from build123d import *

# Parameters (mm, degrees)
SKETCH1_R           = 14
SKETCH1_R_2         = 1.5
BOSS_EXTRUDE1_DEPTH = 8
SKETCH2_W           = 5.1
SKETCH2_H           = 3.455751918
CUT_EXTRUDE2_DEPTH  = 9
CIRPATTERN1_COUNT   = 12
BOSS_EXTRUDE2_START = -4
SKETCH3_R           = 5
SKETCH3_R_2         = 1.5
BOSS_EXTRUDE2_DEPTH = 4


with BuildPart() as part:
    # Sketch1 → Boss-Extrude1 (new body)
    with BuildSketch(Plane.XY):
        Circle(SKETCH1_R)
        Circle(SKETCH1_R_2, mode=Mode.SUBTRACT)
    extrude(amount=BOSS_EXTRUDE1_DEPTH)

    # Sketch2 → Cut-Extrude2 (cut)
    with BuildSketch(Plane.XY):
        with Locations((11.75, 0)):
            Rectangle(SKETCH2_W, SKETCH2_H)
    cut_extrude2 = extrude(amount=CUT_EXTRUDE2_DEPTH, mode=Mode.SUBTRACT)

    # CirPattern1: Cut-Extrude2 ×12 about axis
    cirpattern1_axis = Axis((0, 0, 0), (0, 0, 1))
    for i in range(1, CIRPATTERN1_COUNT):
        add(cut_extrude2.rotate(cirpattern1_axis, i * 360 / CIRPATTERN1_COUNT), mode=Mode.SUBTRACT)

    # Sketch3 → Boss-Extrude2 (add)
    with BuildSketch(Plane.XY.offset(BOSS_EXTRUDE2_START)):
        Circle(SKETCH3_R)
        Circle(SKETCH3_R_2, mode=Mode.SUBTRACT)
    extrude(amount=BOSS_EXTRUDE2_DEPTH)


solid = part.part
Design review of the part built by this model. Coordinates are the model's own, in mm. A direction names the side the tool comes from. Coordinates: 2 decimals unless noted, no trailing zeros. Write each loop counter-clockwise with the first axis right and the second up, starting at its lowest first coordinate (ties: lowest second). Pieces come first, ordered by that corner, then holes. Notation, with made-up numbers: (61, -37.5) - (105, -37.5) arc R9 cw to (105, -31.5) - close; hole circle Ø6 at (88.5, 71). An arc over 180 degrees is marked (long way). One line per item, written item: value.
1) Insertion check: pin 1 (1.7 mm diameter, centred on y = 0, z = 4, fed in from +X); pin 2 (4 mm diameter, centred on x = -0.5, z = 6, fed in from +Y); pin 3 (12 mm diameter, centred on x = 2, y = 8.5, fed in from -Z); pin 4 (1.4 mm diameter, centred on x = -10.5, z = 5, fed in from +Y). Each pin has a flat end and moves straight along its axis. Give the tip position at first contact, or say it passes through.
Answer sheet:
pin 1: stops at x = 9.2
pin 2: stops at y = 13.89
pin 3: stops at z = -4
pin 4: stops at y = 10
2) Add section A-A (y = 0). State the section outline as (x, z) points.
Answer sheet:
outline: (-9.2, 0) - (-5, 0) - (-5, -4) - (-1.5, -4) - (-1.5, 8) - (-9.2, 8) - close; (1.5, -4) - (5, -4) - (5, 0) - (9.2, 0) - (9.2, 8) - (1.5, 8) - close
3) To check wall thickness, follow probe 1 along Y at (x, z) = (4.75, 6.5); probe 2 along Y at (x, z) = (10.5, 3); probe 3 along Y at (x, z) = (5.25, 1.75). State the ranges of each line that lie inside material, in increasing order.
Answer sheet:
probe 1: y = -13.17 to -11.68, -7.88 to 7.88, 11.68 to 13.17
probe 2: y = -9.26 to -8.06, -4.07 to -1.73, 1.73 to 4.07, 8.06 to 9.26
probe 3: y = -12.98 to -12.55, -7.59 to 7.59, 12.55 to 12.98
4) Add section D-D (x = -8). State the section outline as (y, z) points, plus the area to 3 significant figures.
Answer sheet:
outline: (-10.4, 0) - (-6.61, 0) - (-6.61, 8) - (-10.4, 8) - close; (-4.54, 0) - (4.54, 0) - (4.54, 8) - (-4.54, 8) - close; (6.61, 0) - (10.4, 0) - (10.4, 8) - (6.61, 8) - close
area: 133 mm2
5) Add section C-C (y = 4.5). State the section outline as (x, z) points, plus the area to 3 significant figures.
Answer sheet:
outline: (-13.26, 0) - (-11.25, 0) - (-11.25, 8) - (-13.26, 8) - close; (-8.03, 0) - (-2.18, 0) - (-2.18, -4) - (2.18, -4) - (2.18, 0) - (8.03, 0) - (8.03, 8) - (-8.03, 8) - close; (11.25, 0) - (13.26, 0) - (13.26, 8) - (11.25, 8) - close
area: 178 mm2
6) Mouldability with a two-part tool opening along X and no side actions: class faces 6 (the face through (-7.98, -4.58, 3.94)), 7 (the face through (-13.516, 3.65, 3.944)), 8 (the face through (9.107, 7.253, 3.944)) as +X half, -X half, draft (parallel to the pull), parting line (faces both ways), or undercut.
Answer sheet:
face 6: undercut
face 7: -X half
face 8: +X half
7) For faces 1 (the face through (7.955, -4.621, 3.944)), 2 (the face through (1.728, 12, 4)), 3 (the face through (-12, 1.728, 4)), 4 (the face through (12, -1.728, 4)), 5 (the face through (-1.08, -4.88, -2.03)), list the 3-axis set-ups (+Z, -Z, +X, -X, +Y, -Y) from which the entire face can be reached by the end or side of a thin tool; tool diameter is ignored.
Answer sheet:
face 1: +Z, -Z
face 2: +Z, -Z, +Y
face 3: +Z, -Z, -X
face 4: +Z, -Z, +X
face 5: -Z
